Could you check a few things on this drawing? It's one solid part, dimensions in mm from its lowest x, y, z. A direction names the side the tool comes from. Give positions to 0.01 mm unless a question says otherwise; leave off trailing zeros. Write each loop counter-clockwise with the first axis right and the second up, starting at its lowest first coordinate (ties: lowest second). Pieces come first, ordered by that corner, then holes.
1. I'm going to push flat-ended pins straight in: pin 1 (6 mm diameter, centred on y = 114.5, z = 96.5, fed in from -X); pin 2 (5 mm diameter, centred on x = 150, y = 154.5, fed in from +Z). Where does each tip first touch, or does it pass through?
2. Suppose I cut it at A-A (y = 168). Please give me the cut outline in (x, z), and give its area (3 significant figures).
3. If I drill on probe 1 along Z at (x, y) = (69.5, 42); probe 2 along X at (y, z) = (64, 36), over which ranges is the centre line in solid material (lowest first)?
4. Suppose I cut it at B-B (z = 102.5). Please give me the cut outline in (x, y).
5. On a 3-axis mill with a long thin cutter (end or side, diameter ignored), from which of +Z, -Z, +X, -X, +Y, -Y can I reach the whole of each face in a straight line? I mean the marked faces 1, 2 and 3. Say none if no direction works.
6. Suppose I cut it at C-C (x = 40). Please give me the cut outline in (y, z).
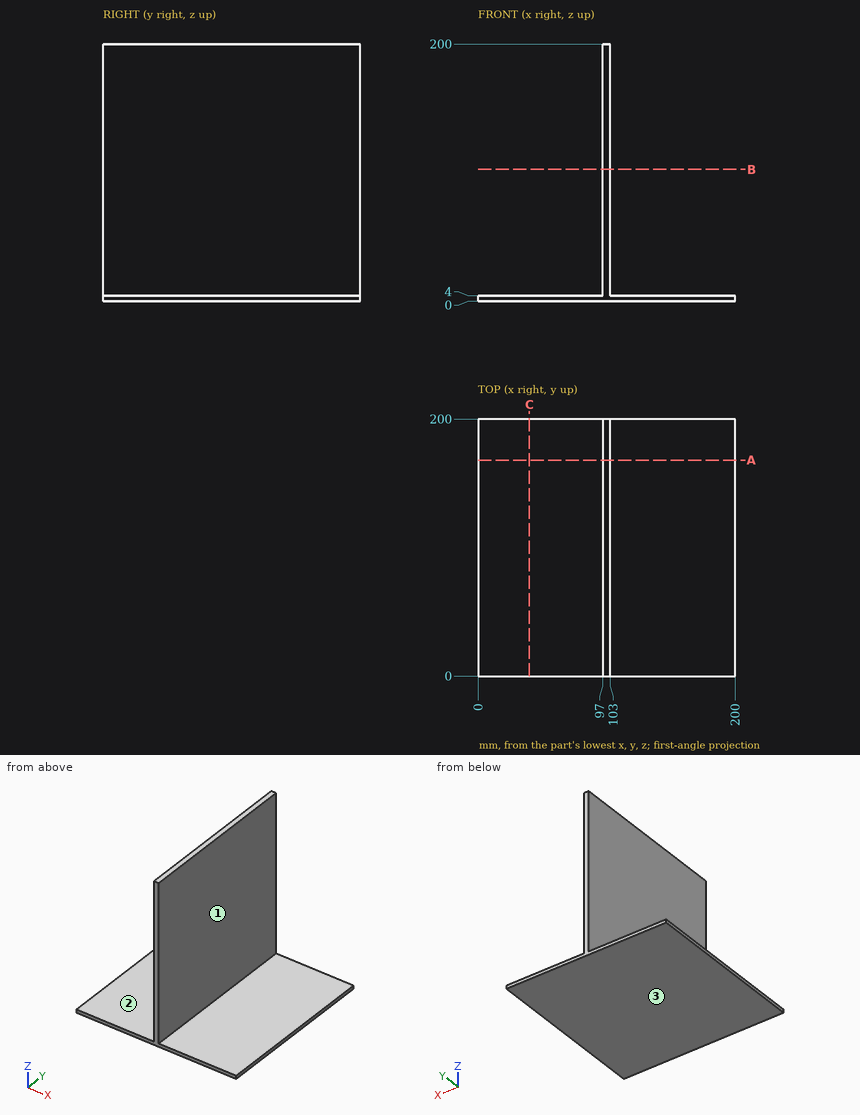
Checks:
1. pin 1: stops at x = 97
1. pin 2: stops at z = 4
2. outline: (0, 0) - (200, 0) - (200, 4) - (103, 4) - (103, 200) - (97, 200) - (97, 4) - (0, 4) - close
2. area: 1,980 mm2
3. probe 1: z = 0 to 4
3. probe 2: x = 97 to 103
4. outline: (97, 0) - (103, 0) - (103, 200) - (97, 200) - close
5. face 1: +Z, +X, +Y, -Y
5. face 2: +Z, -X, +Y, -Y
5. face 3: -Z, +X, -X, +Y, -Y
6. outline: (0, 0) - (200, 0) - (200, 4) - (0, 4) - close
